from build123d import *

# Parameters (mm, degrees)
SKETCH1_R           = 30
BOSS_EXTRUDE1_DEPTH = 85
SKETCH2_R           = 10
CUT_EXTRUDE1_DEPTH  = 85


with BuildPart() as part:
    # Sketch1 → Boss-Extrude1 (new body)
    with BuildSketch(Plane.YZ):
        with BuildLine():
            Line((-165, -83.5), (165, -83.5))
            Line((165, -83.5), (165, -54.5))
            Line((165, -54.5), (103.12562301, -54.5))
            Line((103.12562301, -54.5), (80.090474911, 23.617066466))
            ThreePointArc((80.090474911, 23.617066466), (0, 83.5), (-80.090474911, 23.617066466))
            Line((-80.090474911, 23.617066466), (-103.12562301, -54.5))
            Line((-103.12562301, -54.5), (-165, -54.5))
            Line((-165, -54.5), (-165, -83.5))
        make_face()
        with Locations(Location((0, 1.5, 0), (0, 0, 270))):
            Circle(SKETCH1_R, mode=Mode.SUBTRACT)
    extrude(amount=BOSS_EXTRUDE1_DEPTH)

    # Sketch2 → Cut-Extrude1 (cut)
    with BuildSketch(Plane.XY.offset(-54.5)):
        with Locations((42.5, 125)):
            Circle(SKETCH2_R)
        with Locations(Location((42.5, -125, 0), (0, 0, 270))):
            Circle(SKETCH2_R)
    extrude(amount=-CUT_EXTRUDE1_DEPTH, mode=Mode.SUBTRACT)


solid = part.part
Model file for the job. Use its own axes, mm. A direction names the side the tool comes from. Give positions to 0.01 mm unless a question says otherwise; leave off trailing zeros. Order: outer loops, then holes, each group sorted by start corner. A loop starts at its lowest first (then second) coordinate and runs counter-clockwise, first axis right, second up. Notation, with made-up numbers: (11, -7.75) -> (44, -7.75) arc R13 ccw to (44, 2.25) -> close; hole circle Ø8 at (2, 0.25). An arc over 180 degrees is marked (long way). Use CSV: the item, a comma, the result in double quotes.
1. 3-axis set-ups, long thin cutter, end or side, ignore diameter. For faces 1 (the flat face through (0, -2, -36)), 2 (the flat face through (42, 141, -54.5)), 3 (the flat face through (42, -141, -54.5)): which of +Z, -Z, +X, -X, +Y, -Y reach the whole face in a straight line?
Outcome:
face 1,"+Z, -Z, -X, +Y, -Y"
face 2,"+Z, +X, -X, +Y"
face 3,"+Z, +X, -X, -Y"
2. Band-saw the part on B-B, the plane y = -125. Give the cut face in (x, z).
Outcome:
outline,"(0, -83.5) -> (32.5, -83.5) -> (32.5, -54.5) -> (0, -54.5) -> close; (52.5, -83.5) -> (85, -83.5) -> (85, -54.5) -> (52.5, -54.5) -> close"
3. Drop flat-ended pins along their axis: pin 1 (4 mm diameter, centred on x = 52.5, y = 65, fed in from +Z); pin 2 (8 mm diameter, centred on x = 74, z = -18.5, fed in from -Y); pin 3 (12 mm diameter, centred on x = 72.5, z = 52.5, fed in from -Y). Give the stop position or say it passes through.
Outcome:
pin 1,"z = 54.8"
pin 2,"y = -93.69"
pin 3,"y = -69.35"
4. Mould opens along X. For faces 4 (the flat face through (85, -2, -36)), 5 (the cylindrical face through (32.74, -122.83, -68.8)), 6 (the cylindrical face through (35.13, 131.76, -68.8)), 7 (the cylindrical face through (41.905, 1.501, 83.487)) say: +X half, -X half, draft (parallel to the pull), parting line (faces both ways), or undercut.
Outcome:
face 4,"+X half"
face 5,"undercut"
face 6,"undercut"
face 7,"draft"
5. Band-saw the part on D-D, the plane z = 1.5. Give the cut face in (x, y).
Outcome:
outline,"(0, -86.61) -> (85, -86.61) -> (85, -30) -> (0, -30) -> close; (0, 30) -> (85, 30) -> (85, 86.61) -> (0, 86.61) -> close"
6. Band-saw the part on A-A, the plane x = 42.5. Give the cut face in (y, z), then the cut area to 3 significant figures.
Outcome:
outline,"(-165, -83.5) -> (-135, -83.5) -> (-135, -54.5) -> (-165, -54.5) -> close; (-115, -83.5) -> (115, -83.5) -> (115, -54.5) -> (103.13, -54.5) -> (80.09, 23.62) arc R83.5 ccw to (-80.09, 23.62) -> (-103.13, -54.5) -> (-115, -54.5) -> close; (135, -83.5) -> (165, -83.5) -> (165, -54.5) -> (135, -54.5) -> close; hole circle Ø60 at (0, 1.5)"
area,"27,000 mm²"
7. Band-saw the part on C-C, the plane x = 66. Give the cut face in (y, z), then the cut area to 3 significant figures.
Outcome:
outline,"(-165, -83.5) -> (165, -83.5) -> (165, -54.5) -> (103.13, -54.5) -> (80.09, 23.62) arc R83.5 ccw to (-80.09, 23.62) -> (-103.13, -54.5) -> (-165, -54.5) -> close; hole circle Ø60 at (0, 1.5)"
area,"28,100 mm²"
8. Drill centre lines: line 1 along Y through (x, z) = (42, -75); line 2 along Z through (x, y) = (16.5, -1.5); line 3 along Z through (x, y) = (24, 116.5). Where is each one in solid material? Low to high. Write a range as from..to.
Outcome:
line 1,"-165..-134.99, -115.01..115.01, 134.99..165"
line 2,"-83.5..-28.46, 31.46..83.49"
line 3,"-83.5..-54.5"
